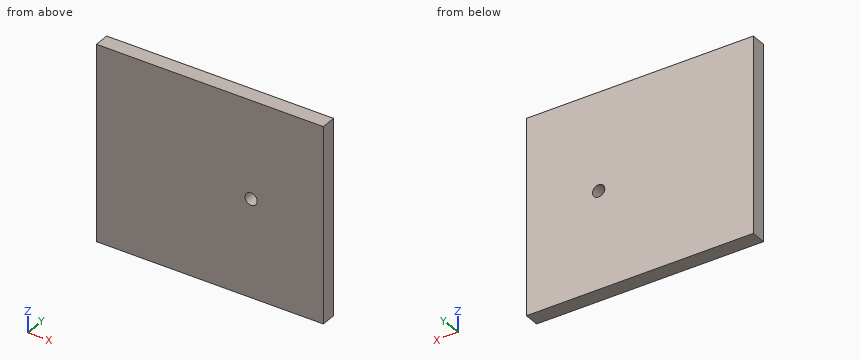
Autodesk Inventor part; units mm, degrees
ref_plane "YZ Plane" through (0, 0, 0) normal (1, 0, 0) x (0, 1, 0)
ref_plane "XZ Plane" through (0, 0, 0) normal (0, 1, 0) x (-1, 0, 0)
ref_plane "XY Plane" through (0, 0, 0) normal (0, 0, 1) x (1, 0, 0)
sketch "Sketch1" plane through (0, 0, 0) normal (0, 1, 0) x (-1, 0, 0)
  line L0 (0, 0) -> (-177.0062, 0)
  line L1 (-177.0062, 0) -> (-177.0062, -152.4)
  line L2 (-177.0062, -152.4) -> (0, -152.4)
  line L3 (0, -152.4) -> (0, 0)
  dimension "d0" = 177.0062
  dimension "d1" = 152.4
extrude "Extrusion1" add sketch "Sketch1" along normal blind 11.9062
sketch "Sketch2" plane through (0, 11.9062, 0) normal (0, 1, 0) x (1, 0, 0)
  line L0 (0, 0) -> (177.0062, 0)
  line L1 (177.0062, 0) -> (177.0062, 152.4)
  line L2 (177.0062, 152.4) -> (0, 152.4)
  line L3 (0, 152.4) -> (0, 0)
  line L4 (0, 0) -> (177.0062, 0)
  line L5 (177.0062, 76.2) -> (120.65, 76.2)
  circle A0 centre (120.65, 76.2) radius 4.7625
  dimension "d4" = 56.3563
  dimension "d5" = 9.525
extrude "Extrusion2" cut sketch "Sketch2" against normal up to surface (11.9062 mm away) contours A0
properties part number "Stage2Wall" material "Wood (Birch)"
Here's how the part is built. I have some questions about the finished solid (model axes, mm). Coordinates: 2 decimals unless noted, no trailing zeros. Order: outer loops, then holes, each group sorted by start corner. A loop starts at its lowest first (then second) coordinate and runs counter-clockwise, first axis right, second up. Notation, with made-up numbers: (-21.75, 20) - (-0.75, 20) arc R25 ccw to (-0.75, 42) - close; hole circle Ø2 at (68, 32). An arc over 180 degrees is marked (long way). Use CSV: the item, a comma, the result in double quotes. Start each with the question number.
1. I'm going to push flat-ended pins straight in: pin 1 (4 mm diameter, centred on y = 5, z = -16.5, fed in from -X); pin 2 (8.5 mm diameter, centred on x = 120.65, z = -76.2, fed in from +Y). Where does each tip first touch, or does it pass through?
2. Suppose I cut it at A-A on z = -76.2. List the corners of the cut face in (x, y) for me.
3. Suppose I cut it at B-B on x = 120.65. List the corners of the cut face in (y, z) for me.
4. Please list where these lines run through material, in increasing order: line 1 (Z direction, x = 120.65, y = 4.5); line 2 (X direction, y = 6.5, z = -76.2); line 3 (X direction, y = 3.25, z = -74). Write a range as from..to.
Output:
1,pin 1,"stops at x = 0"
1,pin 2,"passes through"
2,outline,"(0, 0) - (115.89, 0) - (115.89, 11.91) - (0, 11.91) - close; (125.41, 0) - (177.01, 0) - (177.01, 11.91) - (125.41, 11.91) - close"
3,outline,"(0, -152.4) - (11.91, -152.4) - (11.91, -80.96) - (0, -80.96) - close; (0, -71.44) - (11.91, -71.44) - (11.91, 0) - (0, 0) - close"
4,line 1,"z = -152.4..-80.96, -71.44..0"
4,line 2,"x = 0..115.89, 125.41..177.01"
4,line 3,"x = 0..116.43, 124.87..177.01"
